Part model, mm, in its own coordinate system. Give positions to 0.01 mm unless a question says otherwise; leave off trailing zeros. Write each loop counter-clockwise with the first axis right and the second up, starting at its lowest first coordinate (ties: lowest second). Pieces come first, ordered by that corner, then holes. Notation, with made-up numbers: M 19.5,73 L 55.5,73 A36 cw 55.5,111 Z; hole C 48.25,-31.75 d2. An arc over 180 degrees is marked long. Answer as CSV lines item,"result". Start each with the question number.
Item 1: Band-saw the part on A-A, the plane x = 0. List the corners of the cut face in (y, z).
Item 2: Pin check, flat tip, straight feed: pin 1 (7.5 mm diameter, centred on x = 0, y = 6, fed in from +Z). Stop position of the tip, or through.
Item 3: Wall check: L1, parallel to Y at x = 0, z = 0.8; L2, parallel to Y at x = 3, z = 1.5; L3, parallel to Y at x = 6, z = 1.45. Give the ranges that are in metal, low to high. Write a range as from..to.
Item 4: Two-plate mould, pull along Y, no slides. Class faces 1 (the flat face through (0, 0, 3.1)), 2 (the cylindrical face through (-2.9, 0.98, 1.53)), 3 (the cylindrical face through (-14.985, 0.66, 1.572)): +Y half, -Y half, draft (parallel to the pull), parting line (faces both ways), or undercut.
Item 5: Band-saw the part on C-C, the plane y = -6. List the corners of the cut face in (x, z), then the cut area to 3 significant figures.
Item 6: Band-saw the part on D-D, the plane z = 0.9. List the corners of the cut face in (x, y).
from build123d import *

# Parameters (mm, degrees)
SKETCH1_R           = 12.7
SKETCH1_R_2         = 3.25
BOSS_EXTRUDE1_DEPTH = 3.1
SKETCH2_R           = 15
SKETCH2_R_2         = 12.7
BOSS_EXTRUDE2_DEPTH = 3.1


with BuildPart() as part:
    # Sketch1 → Boss-Extrude1 (new body)
    with BuildSketch(Plane.XY):
        Circle(SKETCH1_R)
        with Locations((-6, 0)):
            Circle(SKETCH1_R_2, mode=Mode.SUBTRACT)
        with Locations((0, 6)):
            Circle(SKETCH1_R_2, mode=Mode.SUBTRACT)
        with Locations((6, 0)):
            Circle(SKETCH1_R_2, mode=Mode.SUBTRACT)
        with Locations((0, -6)):
            Circle(SKETCH1_R_2, mode=Mode.SUBTRACT)
    extrude(amount=BOSS_EXTRUDE1_DEPTH)

    # Sketch2 → Boss-Extrude2 (add, through all)
    with BuildSketch(Plane.XY.offset(3.1)):
        Circle(SKETCH2_R)
        Circle(SKETCH2_R_2, mode=Mode.SUBTRACT)
    extrude(amount=-BOSS_EXTRUDE2_DEPTH)


solid = part.part
Output:
1,outline,"M -15,0 L -9.25,0 L -9.25,3.1 L -15,3.1 Z; M -2.75,0 L 2.75,0 L 2.75,3.1 L -2.75,3.1 Z; M 9.25,0 L 15,0 L 15,3.1 L 9.25,3.1 Z"
2,pin 1,"z = 3.1"
3,L1,"-15..-9.25, -2.75..2.75, 9.25..15"
3,L2,"-14.7..-7.25, -4.75..-1.25, 1.25..4.75, 7.25..14.7"
3,L3,"-13.75..-3.25, 3.25..13.75"
4,face 1,"draft"
4,face 2,"undercut"
4,face 3,"parting line"
5,outline,"M -13.75,0 L -3.25,0 L -3.25,3.1 L -13.75,3.1 Z; M 3.25,0 L 13.75,0 L 13.75,3.1 L 3.25,3.1 Z"
5,area,"65.1 mm²"
6,outline,"C 0,0 d30; hole C -6,0 d6.5; hole C 0,-6 d6.5; hole C 0,6 d6.5; hole C 6,0 d6.5"
